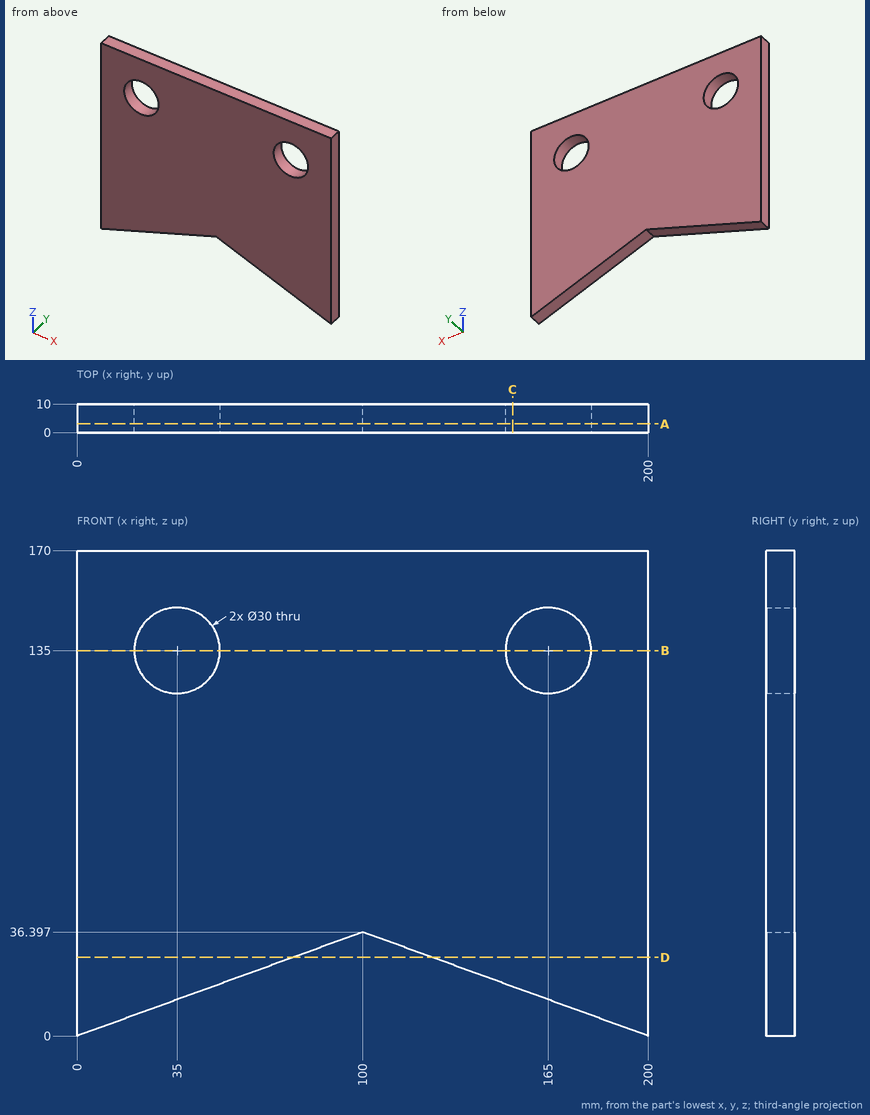
Input: dimensioned drawing with shaded views. Units: mm. Origin: part minimum x, y, z. Coordinates: 2 decimals unless noted, no trailing zeros. Loops run counter-clockwise (first coordinate to the right, second up) from the corner with the lowest first, then second, coordinate; pieces in that order, holes last. Notation, with made-up numbers: (78, 41.5) -> (96, 41.5) arc R36 cw to (96, 76.5) -> close; hole circle Ø1 at (-33.5, 59). An arc over 180 degrees is marked (long way). One line per item, written item: value. Start each with the question number.
Q1. Section query C-C, the plane x = 152.5. Return the cut outline in (y, z), and give its area (3 significant figures).
Q2. Section query D-D, the plane z = 27.5. Return the cut outline in (x, y).
Q3. Section query A-A, the plane y = 3. Return the cut outline in (x, z), and give its area (3 significant figures).
Q4. Line query: line 1 along X through (y, z) = (0.75, 131.5); line 2 along X through (y, z) = (6.75, 143); line 3 along Z through (x, y) = (45.5, 5.5). Output: solid intervals per line, ascending.
Q5. Section query B-B, the plane z = 135. Return the cut outline in (x, y).
Results:
1. outline: (0, 17.29) -> (10, 17.29) -> (10, 126.71) -> (0, 126.71) -> close; (0, 143.29) -> (10, 143.29) -> (10, 170) -> (0, 170) -> close
1. area: 1,360 mm^2
2. outline: (0, 0) -> (75.56, 0) -> (75.56, 10) -> (0, 10) -> close; (124.44, 0) -> (200, 0) -> (200, 10) -> (124.44, 10) -> close
3. outline: (0, 0) -> (100, 36.4) -> (200, 0) -> (200, 170) -> (0, 170) -> close; hole circle Ø30 at (35, 135); hole circle Ø30 at (165, 135)
3. area: 28,900 mm^2
4. line 1: 0 to 20.41, 49.59 to 150.41, 179.59 to 200
4. line 2: 0 to 22.31, 47.69 to 152.31, 177.69 to 200
4. line 3: 16.56 to 124.29, 145.71 to 170
5. outline: (0, 0) -> (20, 0) -> (20, 10) -> (0, 10) -> close; (50, 0) -> (150, 0) -> (150, 10) -> (50, 10) -> close; (180, 0) -> (200, 0) -> (200, 10) -> (180, 10) -> close
